```python
from build123d import *

# Parameters (mm, degrees)
SKETCH1_W           = 40
SKETCH1_H           = 40
BOSS_EXTRUDE1_DEPTH = 14
SKETCH4_W           = 10
SKETCH4_H           = 4
BOSS_EXTRUDE3_DEPTH = 26
SKETCH5_R           = 2
CUT_EXTRUDE2_DEPTH  = 26
SKETCH6_R           = 2.1
CUT_EXTRUDE3_DEPTH  = 15


with BuildPart() as part:
    # Sketch1 → Boss-Extrude1 (new body)
    with BuildSketch(Plane(origin=(0, 0, 0), x_dir=(1, 0, 0), z_dir=(0, 1, 0))):
        with Locations((20, 20)):
            Rectangle(SKETCH1_W, SKETCH1_H)
    extrude(amount=BOSS_EXTRUDE1_DEPTH)

    # Sketch4 → Boss-Extrude3 (add)
    with BuildSketch(Plane(origin=(0, 0, -40), x_dir=(-1, 0, 0), z_dir=(0, 0, -1))):
        with Locations((-20, 12)):
            Rectangle(SKETCH4_W, SKETCH4_H)
    extrude(amount=BOSS_EXTRUDE3_DEPTH)

    # Sketch5 → Cut-Extrude2 (cut)
    with BuildSketch(Plane(origin=(0, 14, 0), x_dir=(1, 0, 0), z_dir=(0, 1, 0))):
        with Locations((20, 60)):
            Circle(SKETCH5_R)
        with Locations((20, 53)):
            Circle(SKETCH5_R)
        with Locations((20, 46)):
            Circle(SKETCH5_R)
    extrude(amount=-CUT_EXTRUDE2_DEPTH, mode=Mode.SUBTRACT)

    # Sketch6 → Cut-Extrude3 (cut, through all)
    with BuildSketch(Plane.XZ):
        with Locations((13, -27)):
            Circle(SKETCH6_R)
        with Locations((20, -27)):
            Circle(SKETCH6_R)
        with Locations((27, -27)):
            Circle(SKETCH6_R)
        with Locations((20, -20)):
            Circle(SKETCH6_R)
        with Locations((27, -20)):
            Circle(SKETCH6_R)
        with Locations((20, -13)):
            Circle(SKETCH6_R)
        with Locations((27, -13)):
            Circle(SKETCH6_R)
        with Locations((13, -20)):
            Circle(SKETCH6_R)
        with Locations((13, -13)):
            Circle(SKETCH6_R)
    extrude(amount=-CUT_EXTRUDE3_DEPTH, mode=Mode.SUBTRACT)


solid = part.part
```
The listing builds one solid part. Answer for the finished solid, in the listing's coordinates (mm). A direction names the side the tool comes from. Give positions to 0.01 mm unless a question says otherwise; leave off trailing zeros. Order: outer loops, then holes, each group sorted by start corner. A loop starts at its lowest first (then second) coordinate and runs counter-clockwise, first axis right, second up. Notation, with made-up numbers: (1.25, -3) -> (49.25, -3) arc R25 ccw to (49.25, 28) -> close; hole circle Ø5 at (26, 37). An arc over 180 degrees is marked (long way). Answer as a JSON object with one key per item and string values. Group by question number.
Item 1: The part is cut by section A-A on z = -46. Write down the section's boundary in (x, y), and give its area (3 significant figures).
Item 2: The part is cut by section C-C on x = 27. Write down the section's boundary in (y, z), and give its area (3 significant figures).
Item 3: The part is cut by section B-B on y = 6.5. Give the number of separate pieces and of enclosed holes in the cut face, and give its area (3 significant figures).
Item 4: A tool of negligible diameter and unlimited length cuts with its end or side. For faces 5 (the flat face through (25, 12, -53)), 6 (the cylindrical face through (20, 12, -62)), 7 (the flat face through (22.3, 10, -52.8)), from which of +Z, -Z, +X, -X, +Y, -Y can it reach the whole face along a straight path? Write none if from no direction.
Item 5: Determine the mould class of faces 1 (the cylindrical face through (26.727, 6.902, -24.918)), 2 (the flat face through (20, 12, -66)), 3 (the flat face through (20, 7, 0)), 4 (the flat face through (15.3, 14, -26.1)) for opening direction Z: pulls with the +Z half, pulls with the -Z half, needs draft (parallel to the pull), parting line crosses it, or undercut.
Item 6: Flat-ended cylindrical pins translate along their axes: pin 1 (3 mm diameter, centred on y = 12.5, z = -49, fed in from -X); pin 2 (3 mm diameter, centred on y = 9, z = -11, fed in from -X); pin 3 (3 mm diameter, centred on y = 12.5, z = -56.5, fed in from +X); pin 4 (6 mm diameter, centred on x = 22.5, y = 2.5, fed in from -Z). Find the tip coordinate at first contact, or state that the pin passes through.
Item 7: Consider L1, parallel to Z at x = 20, y = 7; L2, parallel to Z at x = 35, y = 5.75; L3, parallel to X at y = 11.1, z = -46. Determine where each line is inside the solid, lowest interval first. Write a range as from..to.
Result set:
{
 "1": {"outline": "(15, 10) -> (18, 10) -> (18, 14) -> (15, 14) -> close; (22, 10) -> (25, 10) -> (25, 14) -> (22, 14) -> close", "area": "24.0 mm²"},
 "2": {"outline": "(0, -40) -> (14, -40) -> (14, -29.1) -> (0, -29.1) -> close; (0, -24.9) -> (14, -24.9) -> (14, -22.1) -> (0, -22.1) -> close; (0, -17.9) -> (14, -17.9) -> (14, -15.1) -> (0, -15.1) -> close; (0, -10.9) -> (14, -10.9) -> (14, 0) -> (0, 0) -> close", "area": "384 mm²"},
 "3": {"separate pieces": "1", "enclosed holes": "9", "area": "1,480 mm²"},
 "4": {"face 5": "-Z, +X, +Y, -Y", "face 6": "+Y, -Y", "face 7": "-Z, +X, -X, -Y"},
 "5": {"face 1": "undercut", "face 2": "pulls with the -Z half", "face 3": "pulls with the +Z half", "face 4": "needs draft"},
 "6": {"pin 1": "x = 15", "pin 2": "x = 0", "pin 3": "x = 25", "pin 4": "z = -40"},
 "7": {"L1": "-40..-29.1, -24.9..-22.1, -17.9..-15.1, -10.9..0", "L2": "-40..0", "L3": "15..18, 22..25"}
}
